Design review of the part built by this model. Coordinates are the model's own, in mm. Round coordinates to 2 decimals unless told otherwise and drop trailing zeros. Order: outer loops, then holes, each group sorted by start corner. A loop starts at its lowest first (then second) coordinate and runs counter-clockwise, first axis right, second up. Notation, with made-up numbers: M -17.75,-21 L 28.25,-21 A24 cw 28.25,17 Z; hole C 48,35.5 d3. An arc over 180 degrees is marked long. Write item = value, one per line. Start each with the question number.
```python
from build123d import *

# Parameters (mm, degrees)
F0_W     = 102.382466
F0_H     = 5.877512
F1_DEPTH = 1.016


with BuildPart() as f1:
    # F0 (on Top) → F1 (new body)
    with BuildSketch(Plane.XY):
        with Locations((-51.191233, -2.938756)):
            Rectangle(F0_W, F0_H)
        Polygon((4.706718, 5.804283), (0, 0), (0, -5.877512), (4.706718, -10.5517), (8.460551, -11.758289), (33.664852, -11.758289), (33.664852, -9.479176), (8.460551, -9.479176), (8.460551, -7.200064), (33.664852, -7.200064), (33.664852, -4.518756), (8.460551, -4.518756), (8.460551, -2.105578), (33.664852, -2.105578), (33.664852, 0), (8.460551, 0), (8.460551, 1.78232), (33.664852, 1.78232), (33.664852, 4.195498), (8.460551, 4.195498), (8.460551, 5.804283), (33.664852, 5.804283), (33.664852, 7.94933), (8.460551, 7.94933), align=None)
    extrude(amount=-F1_DEPTH)


solid = f1.part
```
(1) For line 1 along Y through (x, z) = (27, -0.1); line 2 along X through (y, z) = (-2.75, -0.35); line 3 along Y through (x, z) = (-51.5, -0.65), list the stretches that pass through material, from the lowest coordinate up. Write a range as [from, to].
(2) Insertion check: pin 1 (0.5 mm diameter, centred on x = -37.5, z = -0.5, fed in from +Y). The pin has a flat end and moves straight along its axis. Give the tip position at first contact, or say it passes through.
(3) Consider section A-A, the plane x = 18. Write out the cut boundary in (y, z).
(4) Consider section B-B, the plane z = -0.8. Write out the cut boundary in (x, y), then the cut area to 3 significant figures.
(5) Consider section C-C, the plane x = -29. Write out the cut boundary in (y, z), then the cut area to 3 significant figures.
Completed:
q1.line_1 = [-11.76, -9.48], [-7.2, -4.52], [-2.11, 0], [1.78, 4.2], [5.8, 7.95]
q1.line_2 = [-102.38, 8.46]
q1.line_3 = [-5.88, 0]
q2.pin_1 = 0
q3.outline = M -11.76,-1.02 L -9.48,-1.02 L -9.48,0 L -11.76,0 Z; M -7.2,-1.02 L -4.52,-1.02 L -4.52,0 L -7.2,0 Z; M -2.11,-1.02 L 0,-1.02 L 0,0 L -2.11,0 Z; M 1.78,-1.02 L 4.2,-1.02 L 4.2,0 L 1.78,0 Z; M 5.8,-1.02 L 7.95,-1.02 L 7.95,0 L 5.8,0 Z
q4.outline = M -102.38,-5.88 L 0,-5.88 L 4.71,-10.55 L 8.46,-11.76 L 33.66,-11.76 L 33.66,-9.48 L 8.46,-9.48 L 8.46,-7.2 L 33.66,-7.2 L 33.66,-4.52 L 8.46,-4.52 L 8.46,-2.11 L 33.66,-2.11 L 33.66,0 L 8.46,0 L 8.46,1.78 L 33.66,1.78 L 33.66,4.2 L 8.46,4.2 L 8.46,5.8 L 33.66,5.8 L 33.66,7.95 L 8.46,7.95 L 4.71,5.8 L 0,0 L -102.38,0 Z
q4.area = 1,010 mm2
q5.outline = M -5.88,-1.02 L 0,-1.02 L 0,0 L -5.88,0 Z
q5.area = 5.97 mm2
